```python
from build123d import *

# Parameters (mm, degrees)
F0_W     = 105
F0_H     = 90
F1_DEPTH = 3
F3_DEPTH = 16


with BuildPart() as f1:
    # F0 (on Front) → F1 (new body)
    with BuildSketch(Plane.XZ):
        with Locations((-52.5, 45)):
            Rectangle(F0_W, F0_H)
    extrude(amount=F1_DEPTH)

    # F2 (on face) → F3 (join)
    with BuildSketch(Plane.XZ.offset(3)):
        Polygon((0, 0), (0, 90), (-6.666667, 90), (-6.666667, 78), (-14.666667, 78), (-14.666667, 72.5), (-22.666667, 72.5), (-22.666667, 67), (-30.666667, 67), (-30.666667, 59), (-38.666667, 59), (-38.666667, 51), (-46.666667, 51), (-46.666667, 39), (-56.666667, 39), (-56.666667, 29), (-68.666667, 29), (-68.666667, 21), (-84.666667, 21), (-84.666667, 7.5), (-104.666667, 7.5), (-104.666667, 0), align=None)
    extrude(amount=F3_DEPTH)


solid = f1.part
```
Model file for the job. Use its own axes, mm. A direction names the side the tool comes from. Give positions to 0.01 mm unless a question says otherwise; leave off trailing zeros. Loops run counter-clockwise (first coordinate to the right, second up) from the corner with the lowest first, then second, coordinate; pieces in that order, holes last. Notation, with made-up numbers: (23, -3) -> (40, -3) arc R23 cw to (40, 33) -> close; hole circle Ø1 at (-27.75, 6.25). An arc over 180 degrees is marked (long way). Use CSV: the item, a comma, the result in double quotes. Start each with the question number.
1) Slice it at A-A on y = -15.75. Give the cut face in (x, z).
2) Wall check: line 1 (X direction, y = -8.5, z = 38.5); line 2 (Y direction, x = -19, z = 82); line 3 (Z direction, x = -92, y = -12). Give the ranges that are in metal, low to high.
3) Slice it at C-C on z = 41. Give the cut face in (x, y), plus the area to 3 significant figures.
4) Slice it at B-B on x = -49. Give the cut face in (y, z).
5) Tool access for faces 1 (the flat face through (-104.667, -11, 4)), 2 (the flat face through (-105, -1, 44)), 3 (the flat face through (-14.667, -11, 75)): list every direction of +Z, -Z, +X, -X, +Y, -Y with a clear straight run to the whole face (end or side of a thin tool).
6) Flat gauge pins, fed straight in: pin 1 Ø3.5 at (x, y) = (-64, -8.5) entering from +Z; pin 2 Ø1.5 at (x, z) = (-70.5, 32) entering from -Y; pin 3 Ø9.5 at (y, z) = (-13, 43) entering from -X. Where does each tip first touch, or does it go through?
Computed values:
1,outline,"(-104.67, 0) -> (0, 0) -> (0, 90) -> (-6.67, 90) -> (-6.67, 78) -> (-14.67, 78) -> (-14.67, 72.5) -> (-22.67, 72.5) -> (-22.67, 67) -> (-30.67, 67) -> (-30.67, 59) -> (-38.67, 59) -> (-38.67, 51) -> (-46.67, 51) -> (-46.67, 39) -> (-56.67, 39) -> (-56.67, 29) -> (-68.67, 29) -> (-68.67, 21) -> (-84.67, 21) -> (-84.67, 7.5) -> (-104.67, 7.5) -> close"
2,line 1,"x = -56.67 to 0"
2,line 2,"y = -3 to 0"
2,line 3,"z = 0 to 7.5"
3,outline,"(-105, -3) -> (-46.67, -3) -> (-46.67, -19) -> (0, -19) -> (0, 0) -> (-105, 0) -> close"
3,area,"1,060 mm^2"
4,outline,"(-19, 0) -> (0, 0) -> (0, 90) -> (-3, 90) -> (-3, 39) -> (-19, 39) -> close"
5,face 1,"+Z, -Z, -X, -Y"
5,face 2,"+Z, -Z, -X, +Y, -Y"
5,face 3,"+Z, -X, -Y"
6,pin 1,"stops at z = 29"
6,pin 2,"stops at y = -3"
6,pin 3,"stops at x = -56.67"
